```python
from build123d import *

# Parameters (mm, degrees)
ESQUISSE1_W             = 25
ESQUISSE1_H             = 12
BOSS_EXTRU_1_DEPTH      = 10
ESQUISSE2_R             = 4.12
BOSS_EXTRU_2_DEPTH      = 9.5
ESQUISSE3_R             = 2.5
ENL_V_MAT_EXTRU_1_DEPTH = 0.01
ESQUISSE4_R             = 1.75
ENL_V_MAT_EXTRU_2_DEPTH = 15
ESQUISSE5_R             = 1.25
ENL_V_MAT_EXTRU_3_DEPTH = 11
CONG_1_R                = 1
CONG_2_R                = 0.2


with BuildPart() as part:
    # Esquisse1 → Boss.-Extru.1 (new body)
    with BuildSketch(Plane(origin=(0, 0, 0), x_dir=(1, 0, 0), z_dir=(0, 1, 0))):
        with Locations((12.5, 6)):
            Rectangle(ESQUISSE1_W, ESQUISSE1_H)
    extrude(amount=BOSS_EXTRU_1_DEPTH)

    # Esquisse2 → Boss.-Extru.2 (add)
    with BuildSketch(Plane(origin=(0, 10, 0), x_dir=(1, 0, 0), z_dir=(0, 1, 0))):
        with Locations((5, 6)):
            Circle(ESQUISSE2_R)
        with Locations((20, 6)):
            Circle(ESQUISSE2_R)
    extrude(amount=BOSS_EXTRU_2_DEPTH)

    # Esquisse3 → Enlèv. mat.-Extru.1 (cut)
    with BuildSketch(Plane(origin=(0, 19.5, 0), x_dir=(1, 0, 0), z_dir=(0, 1, 0))):
        with Locations((5, 6)):
            Circle(ESQUISSE3_R)
        with Locations((20, 6)):
            Circle(ESQUISSE3_R)
    extrude(amount=-ENL_V_MAT_EXTRU_1_DEPTH, mode=Mode.SUBTRACT)

    # Esquisse4 → Enlèv. mat.-Extru.2 (cut)
    with BuildSketch(Plane(origin=(0, 19.49, 0), x_dir=(1, 0, 0), z_dir=(0, 1, 0))):
        with Locations((5, 6)):
            Circle(ESQUISSE4_R)
        with Locations((20, 6)):
            Circle(ESQUISSE4_R)
    extrude(amount=-ENL_V_MAT_EXTRU_2_DEPTH, mode=Mode.SUBTRACT)

    # Esquisse5 → Enlèv. mat.-Extru.3 (cut, through all)
    with BuildSketch(Plane(origin=(0, 10, 0), x_dir=(1, 0, 0), z_dir=(0, 1, 0))):
        with Locations((12.5, 6)):
            Circle(ESQUISSE5_R)
    extrude(amount=-ENL_V_MAT_EXTRU_3_DEPTH, mode=Mode.SUBTRACT)

    # Congé1
    cong_1_edges = [part.edges().sort_by_distance(p)[0] for p in [
        (0.88, 19.5, -6),
        (15.88, 19.5, -6),
    ]]
    fillet(cong_1_edges, radius=CONG_1_R)

    # Congé2
    cong_2_edges = [part.edges().sort_by_distance(p)[0] for p in [
        (0.88, 10, -6),
        (15.88, 10, -6),
    ]]
    fillet(cong_2_edges, radius=CONG_2_R)


solid = part.part
```
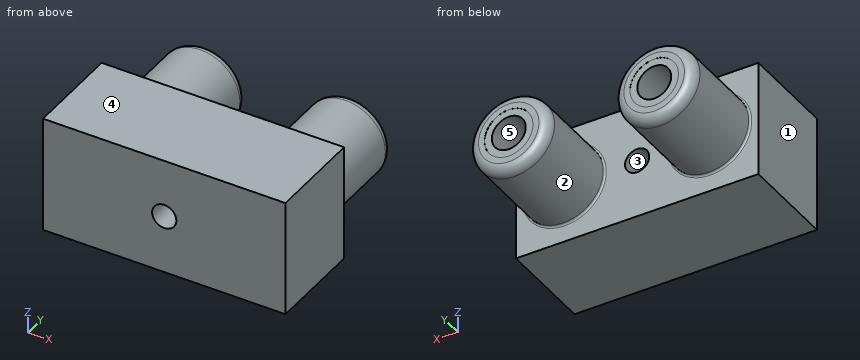
The listing builds one solid part. Answer for the finished solid, in the listing's coordinates (mm). Face numbers are marked on the shaded views. A direction names the side the tool comes from. Give positions to 0.01 mm unless a question says otherwise; leave off trailing zeros. Loops run counter-clockwise (first coordinate to the right, second up) from the corner with the lowest first, then second, coordinate; pieces in that order, holes last. Notation, with made-up numbers: (65, 82) - (106, 82) arc R29 ccw to (106, 105) - close; hole circle Ø7 at (31, 68.25). An arc over 180 degrees is marked (long way). Answer as CSV lines item,"result". Start each with the question number.
Item 1: A cutting plane is placed at C-C on y = 15.75. Determine the outline of the cut face in (x, z), then the cut area to 3 significant figures.
Item 2: Find the intervals of material crossed by line 1 (X direction, y = 11.5, z = -6); line 2 (X direction, y = 2.5, z = -6); line 3 (X direction, y = 18.25, z = -7.25), in increasing order. Write a range as from..to.
Item 3: For the marked faces 4 and 5, determine the directions among +Z, -Z, +X, -X, +Y, -Y from which every point of the face is accessible in a straight line to the end or side of a thin tool.
Item 4: A cutting plane is placed at B-B on x = 12.5. Determine the outline of the cut face in (y, z), then the cut area to 3 significant figures.
Item 5: A cutting plane is placed at A-A on y = 9.25. Determine the outline of the cut face in (x, z).
Item 6: Each of these flat-tipped pins is pushed along its axis until it touches: pin 1 (1.8 mm diameter, centred on x = 4.5, z = -6, fed in from +Y); pin 2 (8 mm diameter, centred on x = 19, y = 15, fed in from -Z); pin 3 (3 mm diameter, centred on x = 20.5, z = -6.5, fed in from +Y). Where does it stop, or does it pass through?
Item 7: The mould has two halves that part along Z. Classify the marked faces 1, 2 and 3: +Z half, -Z half, draft (parallel to the pull), parting line (faces both ways), or undercut.
Found:
1,outline,"circle Ø8.24 at (5, -6); circle Ø8.24 at (20, -6); hole circle Ø3.5 at (5, -6); hole circle Ø3.5 at (20, -6)"
1,area,"87.4 mm^2"
2,line 1,"x = 0.88..3.25, 6.75..9.12, 15.88..18.25, 21.75..24.12"
2,line 2,"x = 0..11.25, 13.75..25"
2,line 3,"x = 1.07..3.78, 6.22..8.93, 16.07..18.78, 21.22..23.93"
3,face 4,"+Z, +X, -X, +Y, -Y"
3,face 5,"+Y"
4,outline,"(0, -12) - (10, -12) - (10, -7.25) - (0, -7.25) - close; (0, -4.75) - (10, -4.75) - (10, 0) - (0, 0) - close"
4,area,"95.0 mm^2"
5,outline,"(0, -12) - (25, -12) - (25, 0) - (0, 0) - close; hole circle Ø3.5 at (5, -6); hole circle Ø2.5 at (12.5, -6); hole circle Ø3.5 at (20, -6)"
6,pin 1,"stops at y = 4.49"
6,pin 2,"stops at z = -10.12"
6,pin 3,"stops at y = 19.49"
7,face 1,"draft"
7,face 2,"parting line"
7,face 3,"undercut"
